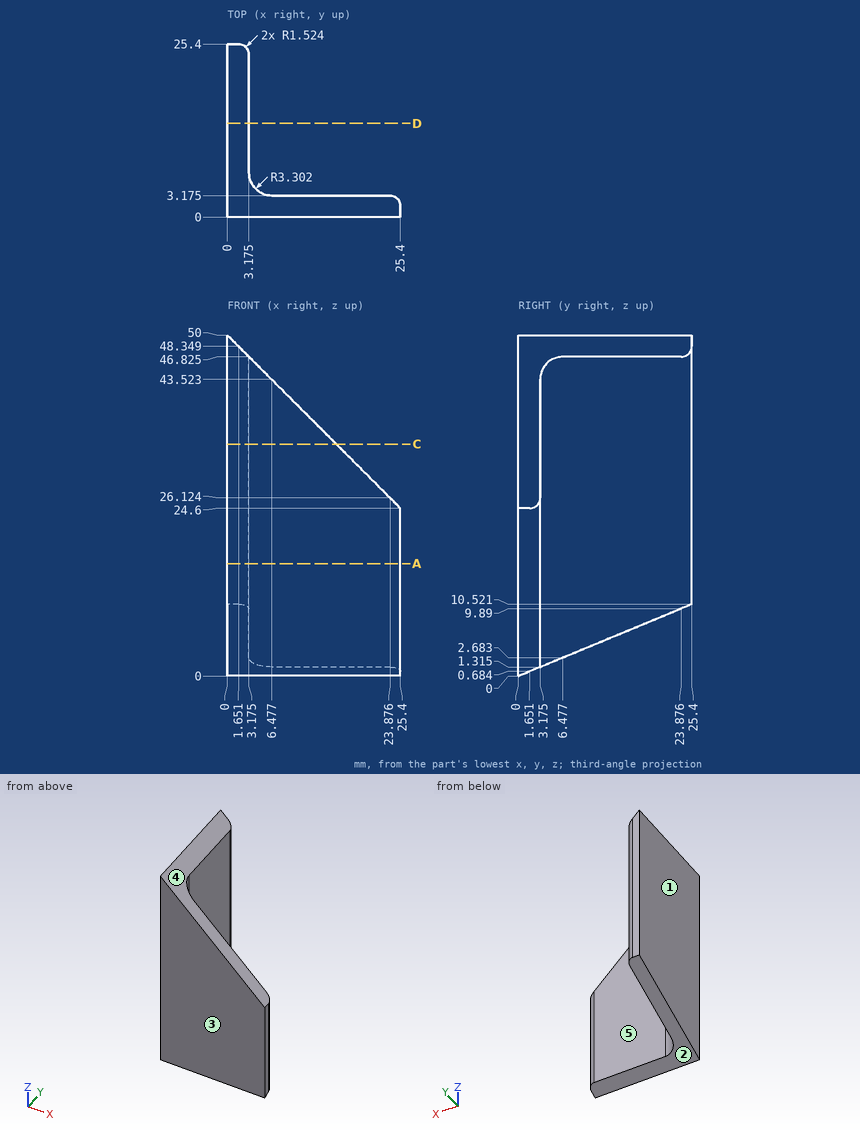
Geometry: see drawing. Coordinates: mm, zero at the bounding-box minimum. A direction names the side the tool comes from. Give positions to 0.01 mm unless a question says otherwise; leave off trailing zeros. Order: outer loops, then holes, each group sorted by start corner. A loop starts at its lowest first (then second) coordinate and runs counter-clockwise, first axis right, second up.
1. Line query: probe 1 along Y at (x, z) = (17.5, 23) (3 decimals); probe 2 along Z at (x, y) = (2.75, 19). Output: solid intervals per line, ascending.
Computed:
probe 1: y = 0 to 3.175
probe 2: z = 7.87 to 47.25
2. Cut plane A-A (z = 16.5). Return loops of the section in (x, y) (3 decimals), and give its area (3 significant figures).
Computed:
outline: (0, 0) - (25.4, 0) - (25.4, 1.651) arc R1.524 ccw to (23.876, 3.175) - (6.477, 3.175) arc R3.302 cw to (3.175, 6.477) - (3.175, 23.876) arc R1.524 ccw to (1.651, 25.4) - (0, 25.4) - close
area: 153 mm2
3. Cut plane C-C (z = 34). Return loops of the section in (x, y) (3 decimals), and give its area (3 significant figures).
Computed:
outline: (0, 0) - (16, 0) - (16, 3.175) - (6.477, 3.175) arc R3.302 cw to (3.175, 6.477) - (3.175, 23.876) arc R1.524 ccw to (1.651, 25.4) - (0, 25.4) - close
area: 123 mm2
4. Pin query (flat end, axial travel): pin 1 Ø5 at (x, z) = (22.5, 16) entering from +Y (3 decimals); pin 2 Ø14 at (y, z) = (14, 20.5) entering from +X (3 decimals). Return the tip coordinate at first contact, or that it passes through.
Computed:
pin 1: stops at y = 3.175
pin 2: stops at x = 3.175
5. Set-up query: the marked faces 4 and 5. Return all of +Z, -Z, +X, -X, +Y, -Y with unobstructed straight access to the full face (end or side cutting, diameter ignored); none if empty.
Computed:
face 4: +Z, +X, +Y, -Y
face 5: +Z, -Z, +X, +Y
6. Draft query along Y for the marked faces 1, 2 and 3. Return one class per face: released by +Y, released by -Y, zero draft, split by the parting line, or undercut.
Computed:
face 1: zero draft
face 2: released by +Y
face 3: released by -Y
7. Cut plane D-D (y = 13.75). Return loops of the section in (x, z) (1 decimal), and give its area (3 significant figures).
Computed:
outline: (0, 5.7) - (3.2, 5.7) - (3.2, 46.8) - (0, 50) - close
area: 136 mm2
